For this review, take the finished solid that the model builds, in its own axes (mm). A direction names the side the tool comes from. Round coordinates to 2 decimals unless told otherwise and drop trailing zeros. Order: outer loops, then holes, each group sorted by start corner. A loop starts at its lowest first (then second) coordinate and runs counter-clockwise, first axis right, second up. Notation, with made-up numbers: M 32,16.5 L 84,16.5 A14 ccw 84,25.5 Z; hole C -28.75,2.5 d8. An arc over 180 degrees is marked long. Use a Markdown table: item, result.
Autodesk Inventor part; units mm, degrees
ref_plane "YZ Plane" through (0, 0, 0) normal (1, 0, 0) x (0, 1, 0)
ref_plane "XZ Plane" through (0, 0, 0) normal (0, 1, 0) x (-1, 0, 0)
ref_plane "XY Plane" through (0, 0, 0) normal (0, 0, 1) x (1, 0, 0)
sketch "Sketch1" plane through (0, 0, 0) normal (0, 1, 0) x (-1, 0, 0)
  line L0 (0, -29.5656) -> (0, 4.9276)
  line L1 (-23.3172, 0) -> (3.8862, 0)
  line L2 (0, 0) -> (-19.431, 0)
  line L3 (-19.431, 0) -> (-19.431, -10.4775)
  line L4 (-19.431, -10.4775) -> (0, -10.4775)
  line L5 (0, -10.4775) -> (0, 0)
  line L6 (0, -10.4775) -> (-12.7, -10.4775)
  line L7 (-12.7, -10.4775) -> (-12.7, -24.638)
  line L8 (0, -24.638) -> (0, -10.4775)
  line L9 (0, -24.638) -> (-12.7, -24.638)
  dimension "d10" = 10.4775
  dimension "d36" = 24.638
  dimension "d37" = 12.7
  dimension "d38" = 19.431
extrude "Extrusion3" add sketch "Sketch1" along normal mid plane 41.91
sketch "Sketch2" plane through (19.431, 20.955, -24.638) normal (0, 0, -1) x (-1, 0, 0)
  line L0 (6.731, -41.91) -> (6.731, 0)
  line L1 (0, 0) -> (6.731, 0)
  line L2 (0, -41.91) -> (0, 0)
  line L3 (6.731, -41.91) -> (0, -41.91)
  line L4 (-3.8862, -20.955) -> (23.3172, -20.955)
  line L5 (19.431, -41.91) -> (19.431, 0)
  point P0 (19.431, -20.955)
  point P1 (5.08, -9.8425)
  point P2 (5.08, -32.0675)
  dimension "d73" = 22.225
  dimension "d74" = 11.1125
  dimension "d75" = 14.351
hole "Hole1" at (14.351, 11.1125, -24.638) at (14.351, -11.1125, -24.638) direction (0, 0, 1) diameter 4.4958 end through all counterbore diameter 8.001 counterbore depth 14.1605
sketch "Sketch3" plane through (0, -20.955, 0) normal (0, 1, 0) x (-1, 0, 0)
  line L0 (-12.7, -24.638) -> (-12.7, -10.4775)
  line L1 (-12.7, -10.4775) -> (-19.431, -10.4775)
  line L2 (-19.431, -10.4775) -> (-12.7, -24.638)
  line L3 (-12.7, -24.638) -> (-12.7, -10.4775)
  line L4 (-19.431, -10.4775) -> (-12.7, -10.4775)
  point P0 (0, 0)
extrude "Extrusion4" add sketch "Sketch3" along normal blind 5.08
sketch "Sketch4" plane through (12.7, 20.955, -24.638) normal (0, 0, -1) x (-1, 0, 0)
  line L0 (12.7, -50.292) -> (12.7, 8.382)
  line L1 (-10.6172, -20.955) -> (16.5862, -20.955)
  line L2 (0, -6.1986) -> (0, 0)
  point P0 (12.7, -20.955)
  point P1 (6.35, -9.525)
  point P2 (6.35, -32.385)
  point P3 (6.35, -20.955)
  point P4 (0, -36.83)
  dimension "d39" = 11.43
  dimension "d40" = 11.43
  dimension "d41" = 6.35
  dimension "d63" = 12.7
hole "Hole2" at (6.35, 11.43, -24.638) at (6.35, -11.43, -24.638) at (6.35, 0, -24.638) direction (0, 0, 1) diameter 2.54 depth 10.922 tip angle 118
sketch "Sketch5" plane through (12.7, 20.955, -10.4775) normal (1, 0, 0) x (0, 0, -1)
  line L0 (-15.4051, -20.955) -> (19.0881, -20.955)
  line L1 (-10.4775, -50.292) -> (-10.4775, 8.382)
  line L2 (6.5405, -12.0396) -> (8.3693, -12.0396)
  line L3 (8.3693, -12.0396) -> (8.3693, -7.0104)
  line L4 (8.3693, -7.0104) -> (6.5405, -7.0104)
  line L5 (6.5405, -7.0104) -> (6.5405, -12.0396)
  line L6 (6.5405, -12.0396) -> (8.3693, -7.0104) construction
  line L7 (8.3693, -12.0396) -> (6.5405, -7.0104) construction
  line L8 (6.5405, -23.4696) -> (8.3693, -23.4696)
  line L9 (8.3693, -23.4696) -> (8.3693, -18.4404)
  line L10 (8.3693, -18.4404) -> (6.5405, -18.4404)
  line L11 (6.5405, -18.4404) -> (6.5405, -23.4696)
  line L12 (6.5405, -23.4696) -> (8.3693, -18.4404) construction
  line L13 (8.3693, -23.4696) -> (6.5405, -18.4404) construction
  line L14 (6.5405, -34.8996) -> (8.3693, -34.8996)
  line L15 (8.3693, -34.8996) -> (8.3693, -29.8704)
  line L16 (8.3693, -29.8704) -> (6.5405, -29.8704)
  line L17 (6.5405, -29.8704) -> (6.5405, -34.8996)
  line L18 (6.5405, -34.8996) -> (8.3693, -29.8704) construction
  line L19 (8.3693, -34.8996) -> (6.5405, -29.8704) construction
  line L20 (14.1605, -6.1986) -> (14.1605, 0)
  point P0 (-10.4775, -20.955)
  point P1 (7.4549, -9.525)
  point P2 (7.4549, -20.955)
  point P3 (7.4549, -32.385)
  point P4 (14.1605, -36.83)
  point P5 (7.4549, -9.525)
  point P6 (7.4549, -32.385)
  dimension "d49" = 5.0292
  dimension "d50" = 1.8288
  dimension "d51" = 11.43
  dimension "d58" = 7.62
  dimension "d59" = 11.43
extrude "Extrusion5" cut sketch "Sketch5" along normal blind 10.16 and the other way blind 9.144
sketch "Sketch6" plane through (0, 20.955, 0) normal (0, 1, 0) x (1, 0, 0)
  line L0 (12.7, 10.4775) -> (12.7, 24.638)
  line L1 (19.431, 10.4775) -> (12.7, 10.4775)
  line L2 (19.431, 10.4775) -> (12.7, 24.638)
  point P0 (0, 0)
extrude "Extrusion6" add sketch "Sketch6" against normal blind 5.08
sketch "Sketch7" plane through (0, 20.955, 0) normal (0, 1, 0) x (1, 0, 0)
  line L0 (0, 0) -> (19.431, 0)
  line L1 (19.431, 0) -> (19.431, 10.4775)
  line L2 (7.7406, 0) -> (19.5357, -3.1605)
  line L3 (19.5357, -3.1605) -> (19.431, 0)
  line L4 (7.7406, 0) -> (19.431, 0)
  dimension "d64" = 11.684
  dimension "d65" = 15
extrude "Extrusion7" [suppressed]
sketch "Sketch8" plane through (19.431, -20.955, 0) normal (1, 0, 0) x (0, 0, -1)
  line L0 (10.4775, 0) -> (10.4775, 5.08)
  line L1 (10.4775, 5.08) -> (10.4775, 36.83)
  line L2 (10.4775, 36.83) -> (10.4775, 41.91)
  line L3 (0, 41.91) -> (10.4775, 41.91)
  line L4 (0, 0) -> (0, 41.91)
  line L5 (10.4775, 0) -> (0, 0)
  line L6 (10.4775, 41.91) -> (-3.81, 41.91)
  line L7 (-3.81, 41.91) -> (-3.81, 0)
  line L8 (-3.81, 0) -> (10.4775, 0)
  line L9 (10.4775, 0) -> (10.4775, 41.91)
  point P0 (0, 20.955)
  dimension "d68" = 0
  dimension "d69" = 3.81
extrude "Extrusion8" [suppressed]
fillet "Fillet2" [suppressed]
equation "\"d23\" = d36 - d10"
Q1. Add section B-B (z = -2). Write out the cut boundary in (x, y) (1 decimal), then the cut area to 3 significant figures.
Determined:
| item | result |
|---|---|
| outline | M 0,-21 L 19.4,-21 L 19.4,21 L 0,21 Z; hole C 14.4,-11.1 d4.5; hole C 14.4,11.1 d4.5 |
| area | 783 mm^2 |
Q2. Add section A-A (y = 9.5). Write out the cut boundary in (x, z).
Determined:
| item | result |
|---|---|
| outline | M 0,-24.64 L 10.69,-24.64 L 10.69,-18.85 L 3.56,-18.85 L 3.56,-17.02 L 10.69,-17.02 L 10.69,-10.48 L 12.78,-10.48 L 12.78,0 L 0,0 Z; M 15.92,-10.48 L 19.43,-10.48 L 19.43,0 L 15.92,0 Z |
Q3. Wall thickness on line 1 along Y through (x, z) = (6.35, -21.75) (3 decimals); line 2 along Z through (x, y) = (6.25, -9.5); line 3 along X through (y, z) = (0, -15.5): over which ranges is each line inside the solid? List them lowest first. Write a range as [from, to].
Determined:
| item | result |
|---|---|
| line 1 | y = [-20.955, -12.7], [-10.16, -1.27], [1.27, 10.16], [12.7, 20.955] |
| line 2 | z = [-24.64, -18.85], [-17.02, 0] |
| line 3 | x = [0, 5.08], [7.62, 12.7] |
Q4. Add section C-C (y = -7). Write out the cut boundary in (x, z).
Determined:
| item | result |
|---|---|
| outline | M 0,-24.64 L 12.7,-24.64 L 12.7,-10.48 L 19.43,-10.48 L 19.43,0 L 0,0 Z |
Q5. Draft analysis for pull direction X (two halves, no side actions). For faces 1 (the flat face through (8, 0, -18.847)), 2 (the flat face through (16.11, 18.45, -17.46)), 3 (the cylindrical face through (15.72, 9.33, -5.17)), 4 (the conical face through (6.13, -0.05, -13.09)), state which applies: pulls with the +X half, pulls with the -X half, needs draft (parallel to the pull), parting line crosses it, or undercut.
Determined:
| item | result |
|---|---|
| face 1 | needs draft |
| face 2 | pulls with the +X half |
| face 3 | undercut |
| face 4 | undercut |
Q6. Machinability: for faces 5 (the cylindrical face through (15.719, -12.896, -5.165)), 6 (the flat face through (10, -20.955, -12)), 7 (the cylindrical face through (7.59, -0.28, -15.34)), 8 (the flat face through (12.7, 0, -19)), 9 (the flat face through (3.556, 0, -18)), which of the approach directions +Z, -Z, +X, -X, +Y, -Y give a long, thin tool a straight path to every point of the face, cutting with its end or side? Answer none if there is none.
Determined:
| item | result |
|---|---|
| face 5 | +Z, -Z |
| face 6 | +Z, -Z, +X, -X, -Y |
| face 7 | -Z |
| face 8 | -Z, +X |
| face 9 | +X |
Q7. Clearance check with flat-ended pins moving along their axes: pin 1 (2 mm diameter, centred on y = -0.5, z = -18, fed in from +X); pin 2 (4 mm diameter, centred on x = 14.35, y = 11.11, fed in from +Z). State where each tip first meets the part, or that it passes through.
Determined:
| item | result |
|---|---|
| pin 1 | stops at x = 12.7 |
| pin 2 | passes through |
